```python
from build123d import *

# Parameters (mm, degrees)
SKETCH1_W           = 151
SKETCH1_H           = 151
BOSS_EXTRUDE1_DEPTH = 25
SKETCH2_W           = 145
SKETCH2_H           = 145
CUT_EXTRUDE1_DEPTH  = 12
SKETCH3_W           = 121
SKETCH3_H           = 6
CUT_EXTRUDE2_DEPTH  = 171.664143862
SKETCH4_W           = 121
SKETCH4_H           = 6
CUT_EXTRUDE3_DEPTH  = 171.664143862
FILLET1_R           = 10
SKETCH5_R           = 3
CUT_EXTRUDE4_DEPTH  = 110.660840777
FILLET4_R           = 2.5
SKETCH6_R           = 1.5
CUT_EXTRUDE5_DEPTH  = 171.664143862


with BuildPart() as part:
    # Sketch1 → Boss-Extrude1 (new body)
    with BuildSketch(Plane(origin=(0, 0, 0), x_dir=(1, 0, 0), z_dir=(0, 1, 0))):
        Rectangle(SKETCH1_W, SKETCH1_H)
    extrude(amount=BOSS_EXTRUDE1_DEPTH)

    # Sketch2 → Cut-Extrude1 (cut)
    with BuildSketch(Plane.XZ):
        Rectangle(SKETCH2_W, SKETCH2_H)
    extrude(amount=-CUT_EXTRUDE1_DEPTH, mode=Mode.SUBTRACT)

    # Sketch3 → Cut-Extrude2 (cut, through all)
    with BuildSketch(Plane.XY.offset(75.5)):
        with Locations((0, 3)):
            Rectangle(SKETCH3_W, SKETCH3_H)
    extrude(amount=-CUT_EXTRUDE2_DEPTH, mode=Mode.SUBTRACT)

    # Sketch4 → Cut-Extrude3 (cut, through all)
    with BuildSketch(Plane.ZY.offset(75.5)):
        with Locations((0, 3)):
            Rectangle(SKETCH4_W, SKETCH4_H)
    extrude(amount=-CUT_EXTRUDE3_DEPTH, mode=Mode.SUBTRACT)

    # Fillet1
    fillet1_edges = [part.edges().sort_by_distance(p)[0] for p in [
        (72.5, 6, 72.5),
        (72.5, 6, -72.5),
        (-72.5, 6, -72.5),
        (-72.5, 6, 72.5),
        (75.5, 12.5, 75.5),
        (-75.5, 12.5, 75.5),
        (-75.5, 12.5, -75.5),
        (75.5, 12.5, -75.5),
    ]]
    fillet(fillet1_edges, radius=FILLET1_R)

    # Sketch5 → Cut-Extrude4 (cut, through all)
    with BuildSketch(Plane(origin=(0, 25, 0), x_dir=(1, 0, 0), z_dir=(0, 1, 0))):
        with Locations(Location((0, 0, 0), (0, 0, 270))):
            Circle(SKETCH5_R)
    extrude(amount=-CUT_EXTRUDE4_DEPTH, mode=Mode.SUBTRACT)

    # Fillet4
    fillet4_edges = [part.edges().sort_by_distance(p)[0] for p in [
        (-60.5, 6, -74),
        (-60.5, 6, 74),
        (60.5, 6, -74),
        (60.5, 6, 74),
        (74, 6, -60.5),
        (-74, 6, -60.5),
        (74, 6, 60.5),
        (-74, 6, 60.5),
    ]]
    fillet(fillet4_edges, radius=FILLET4_R)

    # Sketch6 → Cut-Extrude5 (cut, through all)
    with BuildSketch(Plane(origin=(-75.5, 0, 0), x_dir=(0, 0, -1), z_dir=(1, 0, 0))):
        with Locations(Location((-40, 9, 0), (0, 0, 180))):
            Circle(SKETCH6_R)
        with Locations(Location((40, 9, 0), (0, 0, 180))):
            Circle(SKETCH6_R)
    extrude(amount=CUT_EXTRUDE5_DEPTH, mode=Mode.SUBTRACT)


solid = part.part
```
CAD build for the part. Positions are in the model's coordinates, mm. A direction names the side the tool comes from. Round coordinates to 2 decimals unless told otherwise and drop trailing zeros. Order: outer loops, then holes, each group sorted by start corner. A loop starts at its lowest first (then second) coordinate and runs counter-clockwise, first axis right, second up.
Q1. Which spindle directions (+Z, -Z, +X, -X, +Y, -Y) get a long thin tool onto all of the face, cutting with end or side? Do faces 4 (the flat face through (-1, 9, -72.5)), 5 (the flat face through (-70, 0, 70)). Say none if no direction does.
Q2. Two-plate mould, pull along X, no slides. Class faces 1 (the cylindrical face through (-72.65, 12.68, 72.49)), 2 (the flat face through (75.5, 15, 1)), 3 (the flat face through (-72.5, 9, -1)): pulls with the +X half, pulls with the -X half, needs draft (parallel to the pull), parting line crosses it, or undercut.
Q3. Slice it at B-B (x = 0). Write the cut outline in (y, z), and give its area (3 significant figures).
Q4. Wall check: L1, parallel to Z at x = 49, y = 11.5; L2, parallel to X at y = 22.25, z = 0; L3, parallel to Y at x = 74.15, z = 40. Give the ranges that are in metal, low to high.
Q5. Slice it at C-C (z = -53.5). Write the cut outline in (x, y).
Q6. Drop flat-ended pins along their axis: pin 1 (2.5 mm diameter, centred on x = 8.5, z = 74.5, fed in from -Y); pin 2 (9.5 mm diameter, centred on y = 3, z = -17.5, fed in from -X); pin 3 (3.5 mm diameter, centred on x = 73.5, y = 2.5, fed in from +Z); pin 4 (2.5 mm diameter, centred on x = -74, y = 2, fed in from -Z). Give the stop position or say it passes through.
Q7. Slice it at A-A (z = 0). Write the cut outline in (x, y), and give its area (3 significant figures).
Q8. Slice it at D-D (x = -44.5). Write the cut outline in (y, z), and give its area (3 significant figures).
Results below:
1. face 4: -Y
1. face 5: +Z, -Z, +X, -X, -Y
2. face 1: pulls with the -X half
2. face 2: pulls with the +X half
2. face 3: undercut
3. outline: (6, -75.5) - (25, -75.5) - (25, -3) - (12, -3) - (12, -72.5) - (6, -72.5) - close; (6, 72.5) - (12, 72.5) - (12, 3) - (25, 3) - (25, 75.5) - (6, 75.5) - close
3. area: 1,920 mm2
4. L1: z = -75.5 to -72.5, 72.5 to 75.5
4. L2: x = -75.5 to -3, 3 to 75.5
4. L3: y = 6 to 7.5, 10.5 to 25
5. outline: (-75.5, 6) - (-72.5, 6) - (-72.5, 12) - (72.5, 12) - (72.5, 6) - (75.5, 6) - (75.5, 25) - (-75.5, 25) - close
6. pin 1: stops at y = 6
6. pin 2: stops at x = -75.5
6. pin 3: stops at z = 73.31
6. pin 4: stops at z = -72.39
7. outline: (-75.5, 6) - (-72.5, 6) - (-72.5, 12) - (-3, 12) - (-3, 25) - (-75.5, 25) - close; (3, 12) - (72.5, 12) - (72.5, 6) - (75.5, 6) - (75.5, 25) - (3, 25) - close
7. area: 1,920 mm2
8. outline: (6, -75.5) - (25, -75.5) - (25, 75.5) - (6, 75.5) - (6, 72.5) - (12, 72.5) - (12, -72.5) - (6, -72.5) - close
8. area: 2,000 mm2
